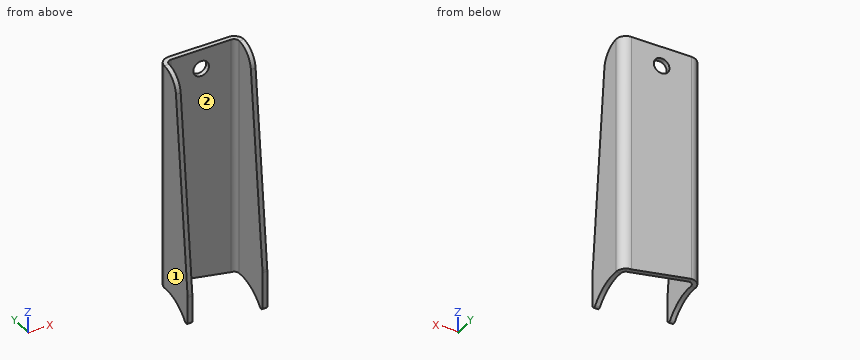
```python
from build123d import *

# Parameters (mm, degrees)
BASE_FLANGE1_START      = -1.4986
BASE_FLANGE1_OUTLINE_W  = 19.05
BASE_FLANGE1_OUTLINE_H  = 95.25
BASE_FLANGE1_DEPTH      = 1.4986
EDGE_FLANGE2_DEPTH      = 95.25
EDGE_FLANGE2_BEND_DEPTH = 95.25
CUT_EXTRUDE2_DEPTH      = 52.76404714123502
CUT_EXTRUDE2_DEPTH_BACK = 52.76404714123502
SKETCH22_R              = 2.4892000000000007
SURFACECUT1_START       = -8.467465696
SURFACECUT1_DEPTH       = 28.142997323
CUT_EXTRUDE5_START      = -7.730915537
CUT_EXTRUDE5_DEPTH      = 7.730915537
CUT_EXTRUDE6_DEPTH      = 3.0988
CUT_EXTRUDE7_DEPTH      = 3.0988
CUT_EXTRUDE3_DEPTH      = 57.19250460256741
FILLET1_R               = 0.79375


# Read off the part's stored shape, not the designer's step: Base-Flange1, SurfaceCut1, Cut-Extrude5
# Sheet-metal steps are written as plain solids
with BuildPart() as part:
    # Base-Flange1 outline → Base-Flange1 (new body)
    with BuildSketch(Plane(origin=(0, 0, 0), x_dir=(1, 0, 0), z_dir=(0, 1, 0)).offset(BASE_FLANGE1_START)):
        Rectangle(BASE_FLANGE1_OUTLINE_W, BASE_FLANGE1_OUTLINE_H)
    extrude(amount=BASE_FLANGE1_DEPTH)

    # Edge-Flange2 section (across the edge) → Edge-Flange2 (add)
    with BuildSketch(Plane(origin=(11.125200000000007, -1.4985999999999888, -47.625), x_dir=(-1, -3.49e-15, 0), z_dir=(0, 0, 1))):
        with BuildLine():
            Line((-1.4985999999999997, 1.6002000000000056), (-1.4985999999999997, 14.3764))
            Line((-1.4985999999999997, 14.3764), (0, 14.3764))
            Line((0, 14.3764), (0, 1.6002000000000056))
            ThreePointArc((0, 1.6002000000000056), (0.46868772874528863, 0.4686877287452902), (1.6002000000000056, 5.55e-15))
            Line((1.6002000000000056, 5.55e-15), (1.600200000000011, -1.4985999999999942))
            ThreePointArc((1.600200000000011, -1.4985999999999942), (-0.5909824935408694, -0.5909824935408718), (-1.4985999999999997, 1.6002000000000056))
        make_face()
    extrude(amount=EDGE_FLANGE2_DEPTH)

    # Edge-Flange2 section 2 (across the edge) → Edge-Flange2 bend (add)
    with BuildSketch(Plane(origin=(-11.125200000000007, -1.4985999999999888, 47.625), x_dir=(1, -3.49e-15, 0), z_dir=(0, 0, -1))):
        with BuildLine():
            Line((-1.4985999999999997, 1.6002000000000056), (-1.4985999999999997, 14.3764))
            Line((-1.4985999999999997, 14.3764), (0, 14.3764))
            Line((0, 14.3764), (0, 1.6002000000000056))
            ThreePointArc((0, 1.6002000000000056), (0.46868772874528863, 0.4686877287452902), (1.6002000000000056, 5.55e-15))
            Line((1.6002000000000056, 5.55e-15), (1.600200000000011, -1.4985999999999942))
            ThreePointArc((1.600200000000011, -1.4985999999999942), (-0.5909824935408694, -0.5909824935408718), (-1.4985999999999997, 1.6002000000000056))
        make_face()
    extrude(amount=EDGE_FLANGE2_BEND_DEPTH)

    # Sketch22 → Cut-Extrude2 (cut, two sides: drawn at the far end of the back side and taken through both)
    with BuildSketch(Plane(origin=(0, 0, 0), x_dir=(1, 0, 0), z_dir=(0, 1, 0)).offset(-CUT_EXTRUDE2_DEPTH_BACK)):
        with Locations(Location((0, -41.275, 0), (0, 0, 270))):
            Circle(SKETCH22_R)
    extrude(amount=CUT_EXTRUDE2_DEPTH + CUT_EXTRUDE2_DEPTH_BACK, mode=Mode.SUBTRACT)

    # SurfaceCut1 outline → SurfaceCut1 (cut)
    with BuildSketch(Plane(origin=(0, 0, 0), x_dir=(0, 1, 0), z_dir=(0.9885166943248128, 0, -0.15111169723467696)).offset(SURFACECUT1_START)):
        with BuildLine():
            ThreePointArc((-4.7625, -28.14850854), (-11.21253157, -29.908348909), (-15.875, -34.700147478))
            Line((-15.875, -34.700147478), (-15.875, -45.396959713))
            Line((-15.875, -45.396959713), (-15.875, -48.985711411))
            Line((-15.875, -48.985711411), (-15.875, -50))
            Line((-15.875, -50), (-1.4986, -50))
            Line((-1.4986, -50), (-1.4986, -48.517446483))
            Line((-1.4986, -48.517446483), (-1.4986, -28.575083721))
            ThreePointArc((-1.4986, -28.575083721), (-3.116671212, -28.255603887), (-4.7625, -28.14850854))
        make_face()
        with BuildLine():
            ThreePointArc((4.904e-06, -29.075295425), (-0.741511706, -28.801863648), (-1.4986, -28.575083721))
            Line((-1.4986, -28.575083721), (-1.4986, -48.517446483))
            Line((-1.4986, -48.517446483), (-1.4986, -50))
            Line((-1.4986, -50), (0, -50))
            Line((0, -50), (0, -48.517446483))
            Line((0, -48.517446483), (4.904e-06, -29.075295425))
        make_face()
    extrude(amount=SURFACECUT1_DEPTH, mode=Mode.SUBTRACT)

    # Cut-Extrude5 outline → Cut-Extrude5 (cut)
    with BuildSketch(Plane(origin=(12.623799999999989, 4.417e-14, 0), x_dir=(0, 0, -1), z_dir=(1, 3.5e-15, 0)).offset(CUT_EXTRUDE5_START)):
        with BuildLine():
            Line((30.161013656, 0), (30.161013656, -3.081973107))
            add(Edge.make_bspline(
                [(30.161013656, -3.081973107), (30.123789076338376, -3.3604465015117064), (30.06785145291286, -3.91981299251284), (30.04917867771754, -4.481604272315385), (30.049178677717507, -5.901493089885278), (30.203533924549607, -7.040390278974325), (30.810097482517182, -9.23799149755241), (31.262254102606217, -10.296510885520753), (32.43252435045563, -12.258659918928036), (33.15053883450323, -13.162125608464567), (34.747119867091556, -14.697775892591103), (35.61176103928939, -15.343862250932757), (36.543461511, -15.875)],
                knots=[7.01e-15, 7.01e-15, 7.01e-15, 7.01e-15, 0.49999999999999956, 1.0000000000000067, 1.0000000000000067, 3.0274304263670744, 3.0274304263670744, 5.054860852734149, 5.054860852734149, 7.082291279101224, 7.082291279101224, 8.9752750105383, 8.9752750105383, 8.9752750105383, 8.9752750105383], degree=3))
            Line((36.543461511, -15.875), (37.033012726, -15.875))
            Line((37.033012726, -15.875), (37.033012726, 0))
            Line((37.033012726, 0), (30.161013656, 0))
        make_face()
    extrude(amount=CUT_EXTRUDE5_DEPTH, mode=Mode.SUBTRACT)

    # Sketch45 → Cut-Extrude6 (cut)
    with BuildSketch(Plane.ZY.offset(12.623799999999989)):
        with BuildLine():
            Line((-27.956993224305993, -3.333e-14), (-30.16101365632842, 9.1e-16))
            Line((-30.16101365632842, 9.1e-16), (-36.543461511337, -8e-16))
            Line((-36.543461511337, -8e-16), (-36.543461511337, -15.874999999986066))
            Line((-36.543461511337, -15.874999999986066), (-33.17348490156023, -15.875000000001156))
            add(Edge.make_bspline(
                [(-33.17348490156023, -15.875000000001156), (-26.545737514477914, -12.250087357596882), (-26.545737514477917, -4.762499999999605)],
                knots=[5.217749490668621, 5.217749490668621, 5.217749490668621, 6.283185307179613, 6.283185307179613, 6.283185307179613], degree=2, weights=[1, 0.8614298921780303, 1]))
            add(Edge.make_bspline(
                [(-26.545737514477917, -4.762499999999605), (-26.54573751447792, -3.9270502006252928), (-26.65645281584444, -3.098800000000031)],
                knots=[2.713e-14, 2.713e-14, 2.713e-14, 0.13137760520102773, 0.13137760520102773, 0.13137760520102773], degree=2, weights=[1, 0.9978432663026745, 1]))
            add(Edge.make_bspline(
                [(-26.65645281584444, -3.098800000000031), (-26.684580856749765, -2.888376912716788), (-26.720679971169147, -2.6830962290480005), (-26.807185378421263, -2.2819272788971268), (-26.85827209747719, -2.08400579105707), (-26.969891004260706, -1.7101957732584916), (-27.030292368751276, -1.5339055104769577), (-27.157879164314696, -1.2013029710556327), (-27.22503599588623, -1.045497343577505), (-27.358398930056477, -0.7651263937563396), (-27.425255566221505, -0.6388233840907098), (-27.556567938722992, -0.41451622077370254), (-27.61948989121088, -0.31919542751514146), (-27.793980163734616, -0.08637757170014503), (-27.892843777023433, -3.459e-14), (-27.956993224305993, -3.333e-14)],
                knots=[0, 0, 0, 0, 0.1249999999999998, 0.1249999999999998, 0.2499999999999996, 0.2499999999999996, 0.37499999999999944, 0.37499999999999944, 0.4999999999999992, 0.4999999999999992, 0.624999999999999, 0.624999999999999, 0.7499999999999989, 0.7499999999999989, 1, 1, 1, 1], degree=3))
        make_face()
    extrude(amount=-CUT_EXTRUDE6_DEPTH, mode=Mode.SUBTRACT)

    # Sketch46 → Cut-Extrude7 (cut)
    with BuildSketch(Plane(origin=(0, 0, 0), x_dir=(1, 0, 0), z_dir=(0, 1, 0))):
        Polygon((-11.125200000000001, 26.65645281584444), (-12.623800000000001, 26.65645281584444), (-12.623800000000044, 30.161013656328407), (9.52499999999999, 30.16101365632841), (-9.525, 26.65645281584444), align=None)
    extrude(amount=-CUT_EXTRUDE7_DEPTH, mode=Mode.SUBTRACT)

    # Sketch36 → Cut-Extrude3 (cut, through all)
    with BuildSketch(Plane.ZY.offset(12.623799999999989)):
        with BuildLine():
            Line((41.90684861578345, -9.493486157833454), (-21.593151384216544, -15.84348615783458))
            ThreePointArc((-21.593151384216544, -15.84348615783458), (-21.908682993060925, -15.867116645973631), (-22.224999999999994, -15.875000000001158))
            Line((-22.224999999999994, -15.875000000001158), (47.625, -15.875000000000039))
            Line((47.625, -15.875000000000039), (47.62499999999999, -3.1750000000000345))
            ThreePointArc((47.62499999999999, -3.1750000000000345), (45.98322358805446, -7.435883786831999), (41.90684861578345, -9.493486157833454))
        make_face()
    extrude(amount=-CUT_EXTRUDE3_DEPTH, mode=Mode.SUBTRACT)

    # Fillet1
    fillet1_edges = [part.edges().sort_by_distance(p)[0] for p in [
        (11.874500000000051, -15.874999999999957, -36.543461511),
        (-11.874500000000051, -15.875000000001114, -33.17348490156023),
    ]]
    fillet(fillet1_edges, radius=FILLET1_R)


solid = part.part
```
Geometry: final body of the model. Coordinates: model frame, mm. Face numbers are marked on the shaded views. A direction names the side the tool comes from. Coordinates: 2 decimals unless noted, no trailing zeros. Write each loop counter-clockwise with the first axis right and the second up, starting at its lowest first coordinate (ties: lowest second). Pieces come first, ordered by that corner, then holes. Notation, with made-up numbers: M 53,56.5 L 69,56.5 A22 ccw 69,82.5 Z; hole C 22.25,86 d5. An arc over 180 degrees is marked long. Answer as CSV lines item,"result". Start each with the question number.
Q1. Cut plane B-B on z = 10.5. Return the cut outline in (x, y) (3 decimals).
Q2. Reachability of the marked faces 1 and 2 from +Z, -Z, +X, -X, +Y, -Y: full face, straight path, thin tool, end or side. Return the list, or none.
Q3. Cut plane D-D on x = -8.5. Return the cut outline in (y, z) (3 decimals).
Q4. Cut plane A-A on x = 0. Return the cut outline in (y, z) (3 decimals), then the cut area to 3 significant figures.
Q5. Line query: line 1 (X direction, y = -12.25, z = 11.5); line 2 (Y direction, x = 9.5, z = -11); line 3 (Z direction, x = 0, y = -1.05) (3 decimals). Output: solid intervals per line, ascending. Write a range as from..to.
Q6. Cut plane C-C on y = -2.25. Return the cut outline in (x, z) (3 decimals).
Q7. Pin query (flat end, axial travel): P1, Ø4, axis at x = 0, z = 41.275, coming from the +Y side; P2, Ø3.5, axis at x = -11.5, y = -2, coming from the -Z side; P3, Ø12, axis at x = -2, z = 7, coming from the -Y side; P4, Ø0.9, axis at x = 11.5, y = -1.5, coming from the -Z side. Return the tip coordinate at first contact, or that it passes through.
Findings below:
1,outline,"M -12.624,-12.634 L -11.125,-12.634 L -11.125,-3.099 A1.6 cw -9.525,-1.499 L 9.525,-1.499 A1.6 cw 11.125,-3.099 L 11.125,-12.634 L 12.624,-12.634 L 12.624,-3.099 A3.099 ccw 9.525,0 L -9.525,0 A3.099 ccw -12.624,-3.099 Z"
2,face 1,"+Z, -Z, -X, +Y, -Y"
2,face 2,"+Z, -Z, -Y"
3,outline,"M -1.499,-26.845 L 0,-26.845 L 0,47.625 L -1.499,47.625 Z"
4,outline,"M -1.499,-28.409 L 0,-28.409 L 0,38.786 L -1.499,38.786 Z; M -1.499,43.764 L 0,43.764 L 0,47.625 L -1.499,47.625 Z"
4,area,"106 mm2"
5,line 1,"x = -12.62..-11.13, 11.13..12.62"
5,line 2,"y = -1.5..0"
5,line 3,"z = -28.409..38.786, 43.764..47.625"
6,outline,"M -12.505,-26.656 L -10.882,-26.656 L -10.882,47.625 L -12.505,47.625 Z; M 10.882,-30.161 L 12.505,-30.161 L 12.505,47.625 L 10.882,47.625 Z"
7,P1,"passes through"
7,P2,"stops at z = -26.66"
7,P3,"stops at y = -1.5"
7,P4,"stops at z = -30.16"
